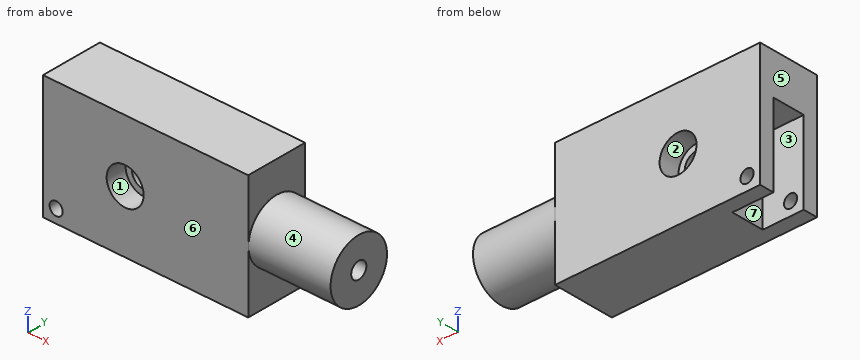
```python
from build123d import *

# Parameters (mm, degrees)
SKETCH1_W           = 25
SKETCH1_H           = 15
BOSS_EXTRUDE1_DEPTH = 7.5
SKETCH2_R           = 3.725
BOSS_EXTRUDE2_DEPTH = 10
SKETCH3_R           = 1
CUT_EXTRUDE1_DEPTH  = 3
SKETCH4_W           = 10
SKETCH4_H           = 4
CUT_EXTRUDE2_DEPTH  = 5
SKETCH5_R           = 0.8
CUT_EXTRUDE3_DEPTH  = 7.5
SKETCH6_R           = 1.5
CUT_EXTRUDE4_DEPTH  = 7.5
SKETCH6_3_R         = 2.25
SKETCH6_3_R_2       = 1.5
CUT_EXTRUDE5_DEPTH  = 2.5
CUT_EXTRUDE6_START  = -2.5
SKETCH7_R           = 2.25
CUT_EXTRUDE6_DEPTH  = 2.5


with BuildPart() as part:
    # Sketch1 → Boss-Extrude1 (new body)
    with BuildSketch(Plane(origin=(0, 0, 0), x_dir=(1, 0, 0), z_dir=(0, 1, 0))):
        with Locations((-9.465160398, -5.033961787)):
            Rectangle(SKETCH1_W, SKETCH1_H)
    extrude(amount=BOSS_EXTRUDE1_DEPTH)

    # Sketch2 → Boss-Extrude2 (add)
    with BuildSketch(Plane(origin=(3.034839602, 0, 0), x_dir=(0, 0, -1), z_dir=(1, 0, 0))):
        with Locations(Location((-5.033961787, 3.75, 0), (0, 0, 180))):
            Circle(SKETCH2_R)
    extrude(amount=BOSS_EXTRUDE2_DEPTH)

    # Sketch3 → Cut-Extrude1 (cut)
    with BuildSketch(Plane(origin=(13.034839602, 0, 0), x_dir=(0, 0, -1), z_dir=(1, 0, 0))):
        with Locations((-5.033961787, 3.75)):
            Circle(SKETCH3_R)
    extrude(amount=-CUT_EXTRUDE1_DEPTH, mode=Mode.SUBTRACT)

    # Sketch4 → Cut-Extrude2 (cut)
    with BuildSketch(Plane.ZY.offset(21.965160398)):
        with Locations((2.533961787, 3.75)):
            Rectangle(SKETCH4_W, SKETCH4_H)
    extrude(amount=-CUT_EXTRUDE2_DEPTH, mode=Mode.SUBTRACT)

    # Sketch5 → Cut-Extrude3 (cut)
    with BuildSketch(Plane(origin=(0, 7.5, 0), x_dir=(1, 0, 0), z_dir=(0, 1, 0))):
        with Locations(Location((-20.365160398, 0.866038213, 0), (0, 0, 270))):
            Circle(SKETCH5_R)
    extrude(amount=-CUT_EXTRUDE3_DEPTH, mode=Mode.SUBTRACT)

    # Sketch6 → Cut-Extrude4 (cut)
    with BuildSketch(Plane(origin=(0, 7.5, 0), x_dir=(1, 0, 0), z_dir=(0, 1, 0))):
        with Locations(Location((-11.965160398, -5.033961787, 0), (0, 0, 270))):
            Circle(SKETCH6_R)
    extrude(amount=-CUT_EXTRUDE4_DEPTH, mode=Mode.SUBTRACT)

    # Sketch6_3 → Cut-Extrude5 (cut)
    with BuildSketch(Plane(origin=(0, 7.5, 0), x_dir=(1, 0, 0), z_dir=(0, 1, 0))):
        with Locations(Location((-11.965160398, -5.033961787, 0), (0, 0, 270))):
            Circle(SKETCH6_3_R)
        with Locations(Location((-11.965160398, -5.033961787, 0), (0, 0, 270))):
            Circle(SKETCH6_3_R_2, mode=Mode.SUBTRACT)
    extrude(amount=-CUT_EXTRUDE5_DEPTH, mode=Mode.SUBTRACT)

    # Sketch7 → Cut-Extrude6 (cut)
    with BuildSketch(Plane.XZ.offset(CUT_EXTRUDE6_START)):
        with Locations(Location((-11.965160398, 5.033961787, 0), (0, 0, 90))):
            Circle(SKETCH7_R)
    extrude(amount=CUT_EXTRUDE6_DEPTH, mode=Mode.SUBTRACT)


solid = part.part
```
Here's how the part is built. I have some questions about the finished solid (model axes, mm). Face numbers are marked on the shaded views. A direction names the side the tool comes from. Coordinates: 2 decimals unless noted, no trailing zeros. Write each loop counter-clockwise with the first axis right and the second up, starting at its lowest first coordinate (ties: lowest second). Pieces come first, ordered by that corner, then holes. Notation, with made-up numbers: M -29,8.5 L -7,8.5 A17 cw -7,28.5 Z; hole C 47.25,78.25 d1. An arc over 180 degrees is marked long. Answer as CSV lines item,"result". Start each with the question number.
Q1. Suppose I cut it at A-A, the plane z = 5.5. List the corners of the cut face in (x, y) for me.
Q2. Will these pins go through, and if not, where does the flat tip stop? pin 1 Ø1.4 at (x, z) = (-20.37, -0.87) entering from +Y; pin 2 Ø4 at (x, z) = (-11.97, 5.03) entering from -Y; pin 3 Ø2.5 at (y, z) = (3.75, 5.03) entering from -X; pin 4 Ø3 at (x, z) = (6.5, 3) entering from -Y.
Q3. I need wall thicknesses on probe 1 along Y at (x, z) = (-19, 4); probe 2 along Z at (x, y) = (-12, 1); probe 3 along X at (y, z) = (4.5, 2.5). Which ranges of each line are inside material? Lowest first, please. Write a range as [from, to].
Q4. For the marked faces 1, 2, 3 and 4, which set-ups out of +Z, -Z, +X, -X, +Y, -Y let a thin tool reach every point of the face, with its end or its side?
Q5. Suppose I cut it at B-B, the plane y = 1. List the corners of the cut face in (x, z) for me, then the cut area to 3 significant figures.
Q6. Suppose I cut it at C-C, the plane x = 6.5. List the corners of the cut face in (y, z) for me (3 decimals), then the cut area to 3 significant figures.
Q7. Suppose I cut it at D-D, the plane y = 3.75. List the corners of the cut face in (x, z) for me.
Q8. If we mould it in two halves opening along Y, with no side actions, what happens to the marked faces 5, 6 and 7? For each: pulls with the +Y half, pulls with the -Y half, needs draft (parallel to the pull), parting line crosses it, or undercut.
Entries:
1,outline,"M -21.97,0 L -14.17,0 L -14.17,2.5 L -13.39,2.5 L -13.39,5 L -14.17,5 L -14.17,7.5 L -21.97,7.5 L -21.97,5.75 L -16.97,5.75 L -16.97,1.75 L -21.97,1.75 Z; M -10.54,2.5 L -9.76,2.5 L -9.76,0 L 3.03,0 L 3.03,0.05 L 13.03,0.05 L 13.03,2.87 L 10.03,2.87 L 10.03,4.63 L 13.03,4.63 L 13.03,7.45 L 3.03,7.45 L 3.03,7.5 L -9.76,7.5 L -9.76,5 L -10.54,5 Z"
2,pin 1,"passes through"
2,pin 2,"stops at y = 2.5"
2,pin 3,"stops at x = -16.97"
2,pin 4,"stops at y = 0.06"
3,probe 1,"y = [0, 1.75], [5.75, 7.5]"
3,probe 2,"z = [-2.47, 2.78], [7.28, 12.53]"
3,probe 3,"x = [-16.97, 13.03]"
4,face 1,"-Y"
4,face 2,"+Y"
4,face 3,"-Z, -X"
4,face 4,"+X"
5,outline,"M -21.97,-2.47 L 3.03,-2.47 L 3.03,2.52 L 13.03,2.52 L 13.03,7.55 L 3.03,7.55 L 3.03,12.53 L -21.97,12.53 Z; hole C -20.37,-0.87 d1.6; hole C -11.97,5.03 d4.5"
5,area,"407 mm²"
6,outline,"C 3.75,5.034 d7.45"
6,area,"43.6 mm²"
7,outline,"M -21.97,7.53 L -16.97,7.53 L -16.97,-2.47 L 3.03,-2.47 L 3.03,1.31 L 13.03,1.31 L 13.03,4.03 L 10.03,4.03 L 10.03,6.03 L 13.03,6.03 L 13.03,8.76 L 3.03,8.76 L 3.03,12.53 L -21.97,12.53 Z; hole C -11.97,5.03 d3"
8,face 5,"needs draft"
8,face 6,"pulls with the -Y half"
8,face 7,"undercut"
